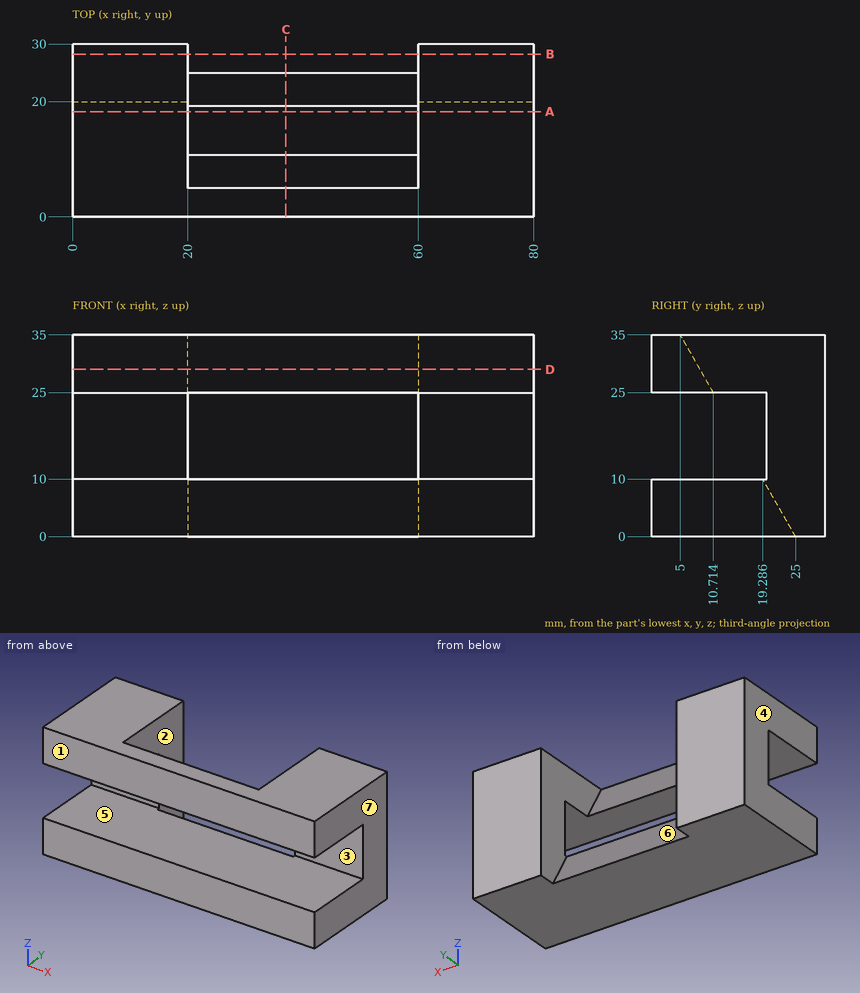
Geometry: see drawing. Coordinates: mm, zero at the bounding-box minimum. A direction names the side the tool comes from. Round coordinates to 2 decimals unless told otherwise and drop trailing zeros. Order: outer loops, then holes, each group sorted by start corner. A loop starts at its lowest first (then second) coordinate and runs counter-clockwise, first axis right, second up. Notation, with made-up numbers: (88, 70.25) -> (100, 70.25) arc R20 cw to (100, 100.25) -> close; hole circle Ø8 at (61, 19.5). An arc over 180 degrees is marked (long way). Write each question's results on one line, items separated by ' | '.
Q1. Ray query, line 1 along Z through (x, y) = (39, 3.5); line 2 along X through (y, z) = (13.75, 33.5); line 3 along Y through (x, z) = (6, 16). Return the intervals inside material, ascending.
Response values:
line 1: 0 to 10, 25 to 35 | line 2: 0 to 20, 60 to 80 | line 3: 20 to 30
Q2. Pin query (flat end, axial travel): pin 1 Ø12 at (y, z) = (26.5, 4) entering from -X; pin 2 Ø12 at (x, z) = (43, 11.5) entering from +Y; pin 3 Ø6 at (x, z) = (21.5, 15.5) entering from -Y; pin 4 Ø6 at (x, z) = (54.5, 27.5) entering from +Y. Return the tip coordinate at first contact, or that it passes through.
Response values:
pin 1: x = 0 | pin 2: y = 21.86 | pin 3: y = 20 | pin 4: y = 10.71
Q3. Access query for the marked faces 1, 2 and 3. Directions: +Z, -Z, +X, -X, +Y, -Y. A direction counts if a zero-diameter tool reaches every point of the face in a straight line with its end or side. Return the directions, or none.
Response values:
face 1: +Z, -Z, +X, -X, -Y | face 2: +Z, +Y | face 3: +X, -X, -Y
Q4. Section query D-D (z = 29). Output: boundary loops of the cut face in (x, y).
Response values:
outline: (0, 0) -> (80, 0) -> (80, 30) -> (60, 30) -> (60, 8.43) -> (20, 8.43) -> (20, 30) -> (0, 30) -> close
Q5. Section query B-B (y = 28.25). Output: boundary loops of the cut face in (x, z).
Response values:
outline: (0, 0) -> (20, 0) -> (20, 35) -> (0, 35) -> close; (60, 0) -> (80, 0) -> (80, 35) -> (60, 35) -> close
Q6. Section query A-A (y = 18.25). Output: boundary loops of the cut face in (x, z).
Response values:
outline: (0, 0) -> (80, 0) -> (80, 10) -> (0, 10) -> close; (0, 25) -> (20, 25) -> (20, 35) -> (0, 35) -> close; (60, 25) -> (80, 25) -> (80, 35) -> (60, 35) -> close
Q7. Pull-direction query (X, two-part tool) for the marked faces 4, 5, 6 and 7; classes: released by +X, released by -X, zero draft, split by the parting line, or undercut.
Response values:
face 4: released by -X | face 5: zero draft | face 6: undercut | face 7: released by +X
Q8. Section query C-C (x = 37). Output: boundary loops of the cut face in (y, z), and give its area (3 significant figures).
Response values:
outline: (0, 0) -> (25, 0) -> (19.29, 10) -> (0, 10) -> close; (0, 25) -> (10.71, 25) -> (5, 35) -> (0, 35) -> close | area: 300 mm²
